from build123d import *

# Parameters (mm, degrees)
SKETCH1_R           = 4.25
BASEHEAD_DEPTH      = 5
SKETCH2_R           = 2.5
BASEBODY_DEPTH      = 12
HEXAGONSOCKET_DEPTH = 2.5
TOPFILLET_R         = 0.625
CHAMFER1_SIZE       = 0.2


with BuildPart() as part:
    # Sketch1 → BaseHead (new body)
    with BuildSketch(Plane(origin=(0, 0, 0), x_dir=(0, 0, -1), z_dir=(1, 0, 0))):
        Circle(SKETCH1_R)
    extrude(amount=BASEHEAD_DEPTH)

    # Sketch2 → BaseBody (add)
    with BuildSketch(Plane(origin=(5, 0, 0), x_dir=(0, 0, -1), z_dir=(1, 0, 0))):
        Circle(SKETCH2_R)
    extrude(amount=BASEBODY_DEPTH)

    # Sketch3 → HexagonSocket (cut)
    with BuildSketch(Plane(origin=(0, 0, 0), x_dir=(0, 0, -1), z_dir=(1, 0, 0))):
        Polygon((2.309401077, 0), (1.154700538, 2), (-1.154700538, 2), (-2.309401077, 0), (-1.154700538, -2), (1.154700538, -2), align=None)
    extrude(amount=HEXAGONSOCKET_DEPTH, mode=Mode.SUBTRACT)

    # Sketch4 → Cut-Revolve1 (revolve, cut)
    with BuildSketch(Plane(origin=(-4.19613823, 0.75, 0), x_dir=(-1, 0, 0), z_dir=(0, 0, 1))):
        Polygon((-6.69613823, 2.75), (-7.850838768, 0.75), (-6.69613823, 0.75), align=None)
    revolve(axis=Axis((0.838992387, 0, 0), (-1, 0, 0)), mode=Mode.SUBTRACT)

    # TopFillet
    topfillet_edges = [part.edges().sort_by_distance(p)[0] for p in [
        (0, 0, 4.25),
    ]]
    fillet(topfillet_edges, radius=TOPFILLET_R)

    # Chamfer1
    chamfer1_edges = [part.edges().sort_by_distance(p)[0] for p in [
        (17, 0, 2.5),
    ]]
    chamfer(chamfer1_edges, length=CHAMFER1_SIZE)


solid = part.part
Design review of the part built by this model. Coordinates are the model's own, in mm. A direction names the side the tool comes from. Coordinates: 2 decimals unless noted, no trailing zeros. Loops run counter-clockwise (first coordinate to the right, second up) from the corner with the lowest first, then second, coordinate; pieces in that order, holes last. Notation, with made-up numbers: (3, 3.5) -> (39, 3.5) arc R18 cw to (39, 17.5) -> close; hole circle Ø6 at (70.25, 56). An arc over 180 degrees is marked (long way). Use a Markdown table: item, result. Add a question column.
Item 1: Wall thickness on L1, parallel to X at y = 2, z = 3; L2, parallel to Z at x = 5.5, y = 1.5; L3, parallel to X at y = 1.25, z = 0: over which ranges is each line inside the solid? List them lowest first. Write a range as from..to.
Item 2: The part is to be moulded in two halves that separate along Y. For faces 1 (the flat face through (1, 2, 0)), 2 (the cylindrical face through (2.782, 3.584, -2.285)), 3 (the flat face through (5, -2, -2)), say which applies: +Y half, -Y half, draft (parallel to the pull), parting line (faces both ways), or undercut.
Item 3: Clearance check with flat-ended pins moving along their axes: P1, Ø4, axis at x = 2, y = -1, coming from the +Z side; P2, Ø0.5, axis at y = -1.5, z = 0.5, coming from the -X side; P3, Ø2, axis at y = 2.5, z = -2.5, coming from the +X side; P4, Ø2, axis at x = 11.5, y = -2.5, coming from the +Z side. State where each tip first meets the part, or that it passes through.
Item 4: We need section A-A, the plane x = 13. Write out the cut boundary in (y, z).
Item 5: Machinability: for faces 4 (the cylindrical face through (10.82, -2.44, 0.54)), 5 (the flat face through (0, -2, -2)), 6 (the flat face through (1.232, 1.014, 1.724)), which of the approach directions +Z, -Z, +X, -X, +Y, -Y give a long, thin tool a straight path to every point of the face, cutting with its end or side? Answer none if there is none.
Numbers:
| question | item | result |
|---|---|---|
| 1 | L1 | x = 0..5 |
| 1 | L2 | z = -2..2 |
| 1 | L3 | x = 2.93..17 |
| 2 | face 1 | undercut |
| 2 | face 2 | parting line |
| 2 | face 3 | draft |
| 3 | P1 | stops at z = 4.25 |
| 3 | P2 | stops at x = 2.6 |
| 3 | P3 | stops at x = 5 |
| 3 | P4 | stops at z = 2 |
| 4 | outline | circle Ø5 at (0, 0) |
| 5 | face 4 | +X |
| 5 | face 5 | +Z, -Z, -X, +Y, -Y |
| 5 | face 6 | -X |
